Geometry check sheet. Reference: the model listing, model coordinates, mm. A direction names the side the tool comes from. Give positions to 0.01 mm unless a question says otherwise; leave off trailing zeros. Loops run counter-clockwise (first coordinate to the right, second up) from the corner with the lowest first, then second, coordinate; pieces in that order, holes last. Notation, with made-up numbers: (21, 34.25) -> (69, 34.25) arc R30 ccw to (69, 63.25) -> close; hole circle Ø9 at (46, 80.25). An arc over 180 degrees is marked (long way). Write each question's results on one line, items separated by ' | '. Start each with the question number.
1) Sectioned sample at D-D on x = -30.5. Record the cut outline in (y, z), then the cut area to 3 significant figures.
2) Depth check by flat-ended pin: pin 1 (1 mm diameter, centred on x = -0.5, z = 11, fed in from +Y); pin 2 (5 mm diameter, centred on x = 26, z = -9, fed in from -Y); pin 3 (12 mm diameter, centred on y = 32.5, z = -17.5, fed in from +X); pin 4 (11.5 mm diameter, centred on x = 0, z = 0, fed in from -Y). Enter the tip coordinate at first touch or a pass-through.
3) Draft check along Z on faces 1 (the face through (6, 20, -1.25)), 2 (the face through (6, 20, 1.25)), 3 (the face through (-5.077, 19.72, -38.668)), 4 (the face through (8, 40, 8)). Enter one of: pulls with the +Z half, pulls with the -Z half, needs draft (parallel to the pull), parting line crosses it, or undercut.
4) Sectioned sample at A-A on x = 0. Record the cut outline in (y, z), then the cut area to 3 significant figures.
5) Scan lines: line 1 (Z direction, x = 0, y = 15); line 2 (X direction, y = 22.5, z = 0); line 3 (Y direction, x = -27.5, z = 1). Record each from-to range of solid material in increasing order. Write a range as from..to.
6) Set-up check for faces 5 (the face through (-2.17, 40.99, 9.76)), 6 (the face through (7.5, 20, 0)), 7 (the face through (-5, -2, 2)), 8 (the face through (-2.17, -0.99, 9.76)): record each of +Z, -Z, +X, -X, +Y, -Y from which the full face is reachable in a straight line by a thin tool's end or side.
7) Sectioned sample at C-C on y = 14.5. Record the cut outline in (x, z), then the cut area to 3 significant figures.
8) Sectioned sample at B-B on z = 0. Record the cut outline in (x, y).
```python
from build123d import *

# Parameters (mm, degrees)
SKETCH1_R                = 39
BOSS_EXTRUDE1_DEPTH      = 40
SKETCH2_R                = 10
BOSS_EXTRUDE2_DEPTH      = 2
BOSS_EXTRUDE2_DEPTH_BACK = 42
SKETCH3_R                = 5
CUT_EXTRUDE1_DEPTH       = 1
CUT_EXTRUDE1_DEPTH_BACK  = 45
SKETCH4_W                = 5
SKETCH4_H                = 2.5
CUT_EXTRUDE2_DEPTH       = 45


with BuildPart() as part:
    # Sketch1 → Boss-Extrude1 (new body)
    with BuildSketch(Plane(origin=(0, 0, 0), x_dir=(1, 0, 0), z_dir=(0, 1, 0))):
        Circle(SKETCH1_R)
    extrude(amount=BOSS_EXTRUDE1_DEPTH)

    # Sketch2 → Boss-Extrude2 (add, two sides)
    with BuildSketch(Plane(origin=(0, 40, 0), x_dir=(1, 0, 0), z_dir=(0, 1, 0))) as boss_extrude2_sk:
        Circle(SKETCH2_R)
    extrude(amount=BOSS_EXTRUDE2_DEPTH)
    extrude(boss_extrude2_sk.sketch, amount=-BOSS_EXTRUDE2_DEPTH_BACK)

    # Sketch3 → Cut-Extrude1 (cut, two sides)
    with BuildSketch(Plane(origin=(0, 42, 0), x_dir=(1, 0, 0), z_dir=(0, 1, 0))) as cut_extrude1_sk:
        Circle(SKETCH3_R)
    extrude(amount=CUT_EXTRUDE1_DEPTH, mode=Mode.SUBTRACT)
    extrude(cut_extrude1_sk.sketch, amount=-CUT_EXTRUDE1_DEPTH_BACK, mode=Mode.SUBTRACT)

    # Sketch4 → Cut-Extrude2 (cut, through all)
    with BuildSketch(Plane(origin=(0, 42, 0), x_dir=(1, 0, 0), z_dir=(0, 1, 0))):
        with Locations((5, 0)):
            Rectangle(SKETCH4_W, SKETCH4_H)
    extrude(amount=-CUT_EXTRUDE2_DEPTH, mode=Mode.SUBTRACT)


solid = part.part
```
Result:
1) outline: (0, -24.31) -> (40, -24.31) -> (40, 24.31) -> (0, 24.31) -> close | area: 1,940 mm^2
2) pin 1: y = 40 | pin 2: y = 0 | pin 3: x = 37.27 | pin 4: y = -2
3) face 1: undercut | face 2: undercut | face 3: parting line crosses it | face 4: needs draft
4) outline: (-2, -10) -> (0, -10) -> (0, -39) -> (40, -39) -> (40, -10) -> (42, -10) -> (42, -5) -> (-2, -5) -> close; (-2, 5) -> (42, 5) -> (42, 10) -> (40, 10) -> (40, 39) -> (0, 39) -> (0, 10) -> (-2, 10) -> close | area: 2,760 mm^2
5) line 1: -39..-5, 5..39 | line 2: -39..-5, 7.5..39 | line 3: 0..40
6) face 5: +Y | face 6: +Y, -Y | face 7: +Z, -Z, +X, -X, -Y | face 8: -Y
7) outline: circle Ø78 at (0, 0); hole (4.84, -1.25) -> (7.5, -1.25) -> (7.5, 1.25) -> (4.84, 1.25) arc R5 ccw (long way) to start | area: 4,690 mm^2
8) outline: (-39, 0) -> (-10, 0) -> (-10, -2) -> (-5, -2) -> (-5, 42) -> (-10, 42) -> (-10, 40) -> (-39, 40) -> close; (7.5, -2) -> (10, -2) -> (10, 0) -> (39, 0) -> (39, 40) -> (10, 40) -> (10, 42) -> (7.5, 42) -> close
